```python
from build123d import *

# Parameters (mm, degrees)
BOSS_EXTRUDE1_DEPTH = 3
CIRPATTERN1_COUNT   = 15
SKETCH2_R           = 12.73044952
BOSS_EXTRUDE2_DEPTH = 2.54


with BuildPart() as part:
    # Sketch1 → Boss-Extrude1 (new body, symmetric)
    with BuildSketch(Plane(origin=(0, 0, 0), x_dir=(1, 0, 0), z_dir=(0, 1, 0))):
        with BuildLine():
            ThreePointArc((0, 9.305199576), (1.058591657, 9.732470692), (1.52399559, 10.774860293))
            ThreePointArc((1.52399559, 10.774860293), (1.684189321, 11.094304623), (2.030537225, 11.182337802))
            ThreePointArc((2.030537225, 11.182337802), (2.362957849, 11.116842642), (2.693278481, 11.041467799))
            ThreePointArc((2.693278481, 11.041467799), (2.973876716, 10.820173105), (2.990291257, 10.463189528))
            ThreePointArc((2.990291257, 10.463189528), (2.991480859, 9.321622409), (3.784765639, 8.500722805))
            ThreePointArc((3.784765639, 8.500722805), (-1.934659777, -9.10185864), (0, 9.305199576))
        make_face()
    boss_extrude1 = extrude(amount=BOSS_EXTRUDE1_DEPTH, both=True)

    # CirPattern1: Boss-Extrude1 ×15 about axis
    cirpattern1_axis = Axis((0, 0, 0), (0, 1, 0))
    for i in range(1, CIRPATTERN1_COUNT):
        add(boss_extrude1.rotate(cirpattern1_axis, i * 360 / CIRPATTERN1_COUNT))

    # Sketch2 → Boss-Extrude2 (add)
    with BuildSketch(Plane.XZ.offset(3)):
        Circle(SKETCH2_R)
    extrude(amount=BOSS_EXTRUDE2_DEPTH)


solid = part.part
```
Geometry: final body of the model. Coordinates: model frame, mm. A direction names the side the tool comes from. Round coordinates to 2 decimals unless told otherwise and drop trailing zeros. Order: outer loops, then holes, each group sorted by start corner. A loop starts at its lowest first (then second) coordinate and runs counter-clockwise, first axis right, second up. Notation, with made-up numbers: (16, 43.5) -> (42, 43.5) arc R24 ccw to (42, 68.5) -> close; hole circle Ø5 at (79.25, 24.5). An arc over 180 degrees is marked (long way). Use one line per item in the form item = value. Start each with the question number.
1. Reachability of faces 1 (the face through (5.874, -4.252, -11.294)), 2 (the face through (-6, -3, 8)) from +Z, -Z, +X, -X, +Y, -Y: full face, straight path, thin tool, end or side. Return the list, or none.
2. Pin query (flat end, axial travel): pin 1 Ø5 at (y, z) = (-3, -8) entering from +X; pin 2 Ø2 at (x, y) = (-9, -1) entering from -Z; pin 3 Ø4 at (y, z) = (-2.5, 1.5) entering from +X; pin 4 Ø2 at (x, y) = (-9, -3.5) entering from +Z. Return the tip coordinate at first contact, or that it passes through.
3. Line query: probe 1 along Y at (x, z) = (6, -9.75); probe 2 along Z at (x, y) = (0.25, -4); probe 3 along Z at (x, y) = (-8.25, 2.75). Output: solid intervals per line, ascending.
4. Cut plane A-A (z = -2.5). Return the cut outline in (x, y), then the cut area to 3 significant figures.
Solution:
q1.face_1 = +Y, -Y
q1.face_2 = +Y
q2.pin_1 = 11.48
q2.pin_2 = -6.18
q2.pin_3 = 12.73
q2.pin_4 = 9.9
q3.probe_1 = -5.54 to -3
q3.probe_2 = -12.73 to 12.73
q3.probe_3 = -5.74 to 4.39, 6.44 to 7.82
q4.outline = (-12.48, -5.54) -> (12.48, -5.54) -> (12.48, -3) -> (9.03, -3) -> (9.03, 3) -> (-9.03, 3) -> (-9.03, -3) -> (-12.48, -3) -> close
q4.area = 172 mm^2
